Can you work these out from the model? Positions are in its coordinate system, mm. Face numbers are marked on the shaded views. A direction names the side the tool comes from. Coordinates: 2 decimals unless noted, no trailing zeros. Order: outer loops, then holes, each group sorted by start corner. A loop starts at its lowest first (then second) coordinate and runs counter-clockwise, first axis right, second up. Notation, with made-up numbers: (-16, 65.5) -> (23, 65.5) arc R4 cw to (23, 71.5) -> close; hole circle Ø7 at (42.5, 69). An arc over 180 degrees is marked (long way). Answer as a JSON object with one key per item and string values. Group by question number.
(1) For pin 1 (3 mm diameter, centred on y = 1.5, z = 14.5, fed in from -X); pin 2 (4 mm diameter, centred on x = -0.5, y = 2, fed in from -Z); pin 3 (2 mm diameter, centred on x = 2, z = 35, fed in from -Y); pin 4 (1.5 mm diameter, centred on y = -2, z = 33, fed in from -X), each with a flat end and sliding along its axis, tell me the tip position at first contact or that it passes through.
(2) Which directions (+Z, -Z, +X, -X, +Y, -Y) give clear straight access to the entire face, cutting with the end or side of a thin tool? Please do the marked faces 1 and 2.
(3) I want a section at A-A, the plane x = 0. List the corners of the cut face in (y, z) for me, plus the area to 3 significant figures.
(4) I want a section at D-D, the plane z = 23.5. List the corners of the cut face in (x, y) for me, plus the area to 3 significant figures.
(5) I need wall thicknesses on line 1 (X direction, y = -2.5, z = 11.5); line 2 (X direction, y = -0.75, z = 35); line 3 (Z direction, x = -0.75, y = 0.5). Which ranges of each line are inside material? Lowest first, please.
(6) I want a section at C-C, the plane z = 5. List the corners of the cut face in (x, y) for me, plus the area to 3 significant figures.
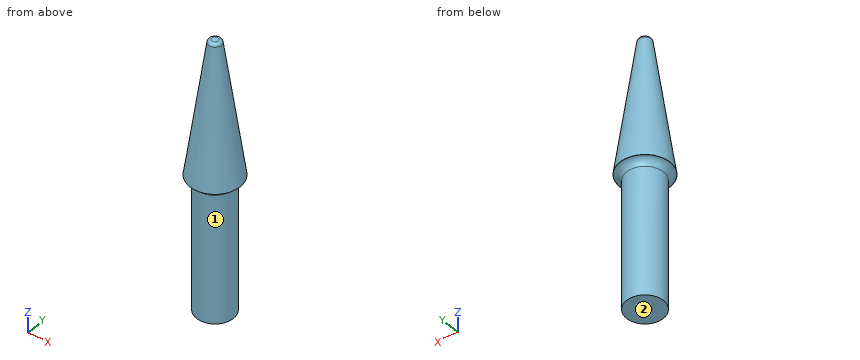
from build123d import *


with BuildPart() as f1:
    # F0 (on Front) → F1 (revolve)
    with BuildSketch(Plane.XZ):
        with BuildLine():
            Line((3.9, 21), (0.995087, 41.569917))
            ThreePointArc((0.995087, 41.569917), (0.827904, 41.877464), (0.5, 42))
            Line((0.5, 42), (0, 42))
            Line((0, 42), (0, 0))
            Line((0, 0), (2.85, 0))
            Line((2.85, 0), (2.85, 20))
            ThreePointArc((2.85, 20), (3.142893, 20.707107), (3.85, 21))
            Line((3.85, 21), (3.9, 21))
        make_face()
    revolve(axis=Axis((0, 0, 21), (0, 0, 1)))


solid = f1.part
Computed values:
{
 "1": {"pin 1": "stops at x = -2.85", "pin 2": "stops at z = 0", "pin 3": "stops at y = -1.66", "pin 4": "stops at x = -1.83"},
 "2": {"face 1": "-Z", "face 2": "-Z, +X, -X, +Y, -Y"},
 "3": {"outline": "(-3.9, 21) -> (-3.85, 21) arc R1 cw to (-2.85, 20) -> (-2.85, 0) -> (2.85, 0) -> (2.85, 20) arc R1 cw to (3.85, 21) -> (3.9, 21) -> (1, 41.57) arc R0.5 ccw to (0.5, 42) -> (-0.5, 42) arc R0.5 ccw to (-1, 41.57) -> close", "area": "222 mm2"},
 "4": {"outline": "circle Ø7.09 at (0, 0)", "area": "39.5 mm2"},
 "5": {"line 1": "x = -1.37 to 1.37", "line 2": "x = -1.77 to 1.77", "line 3": "z = 0 to 41.8"},
 "6": {"outline": "circle Ø5.7 at (0, 0)", "area": "25.5 mm2"}
}
